```python
from build123d import *

# Parameters (mm, degrees)
SKETCH1_W           = 35
SKETCH1_H           = 10.4
BOSS_EXTRUDE1_DEPTH = 1
BOSS_EXTRUDE3_DEPTH = 3
SKETCH3_W           = 3.5
SKETCH3_H           = 8.5
BOSS_EXTRUDE4_DEPTH = 1.2


with BuildPart() as part:
    # Sketch1 → Boss-Extrude1 (new body)
    with BuildSketch(Plane.XY):
        Rectangle(SKETCH1_W, SKETCH1_H)
    extrude(amount=BOSS_EXTRUDE1_DEPTH)

    # Sketch2 → Boss-Extrude3 (add)
    with BuildSketch(Plane.XY.offset(1)):
        with BuildLine():
            Line((15.253902663, 2.079032558), (10.253902663, 2.079032558))
            ThreePointArc((10.253902663, 2.079032558), (9.003902663, 3.329032558), (10.253902663, 4.579032558))
            Line((10.253902663, 4.579032558), (15.253902663, 4.579032558))
            ThreePointArc((15.253902663, 4.579032558), (16.503902663, 3.329032558), (15.253902663, 2.079032558))
        make_face()
    extrude(amount=BOSS_EXTRUDE3_DEPTH)

    # Sketch3 → Boss-Extrude4 (add)
    with BuildSketch(Plane.XY.offset(1)):
        with Locations((-1.547221583, 0.122630604)):
            Rectangle(SKETCH3_W, SKETCH3_H)
    extrude(amount=BOSS_EXTRUDE4_DEPTH)


solid = part.part
```
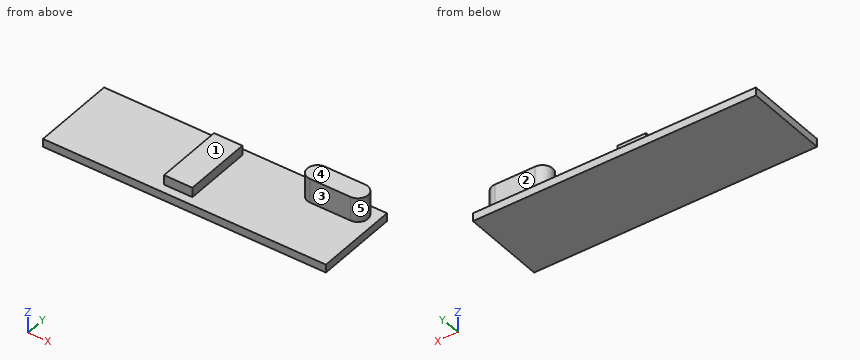
CAD build for the part. Positions are in the model's coordinates, mm. Face numbers are marked on the shaded views. A direction names the side the tool comes from. Round coordinates to 2 decimals unless told otherwise and drop trailing zeros. Write each loop counter-clockwise with the first axis right and the second up, starting at its lowest first coordinate (ties: lowest second). Pieces come first, ordered by that corner, then holes. Notation, with made-up numbers: (60, 38) -> (108, 38) arc R12 ccw to (108, 42) -> close; hole circle Ø7 at (70.5, -13.5). An arc over 180 degrees is marked (long way). Answer in a Markdown table with one row per item. Add a question column.
Item 1: Saw through at C-C, the plane x = 6. Write the cut outline in (y, z), then the cut area to 3 significant figures.
Item 2: Saw through at A-A, the plane z = 1.45. Write the cut outline in (x, y).
Item 3: Saw through at D-D, the plane z = 3.25. Write the cut outline in (x, y), then the cut area to 3 significant figures.
Item 4: Which spindle directions (+Z, -Z, +X, -X, +Y, -Y) get a long thin tool onto all of the face, cutting with end or side? Do the marked faces 1, 2, 3, 4 and 5. Say none if no direction does.
Item 5: Drill centre lines: line 1 (X direction, y = -3.25, z = 1.6); line 2 (Z direction, x = 6, y = 1); line 3 (Y direction, x = 10.5, z = 3.1). Where is each one in solid material? Low to high. Write a range as from..to.
Item 6: Saw through at B-B, the plane y = 0.75. Write the cut outline in (x, z).
Item 7: Drop flat-ended pins along their axis: pin 1 Ø3 at (x, y) = (5.5, 0.5) entering from +Z; pin 2 Ø1 at (x, z) = (-2, 2) entering from -Y; pin 3 Ø0.6 at (y, z) = (2, 1.5) entering from -X. Give the stop position or say it passes through.
Findings below:
| question | item | result |
|---|---|---|
| 1 | outline | (-5.2, 0) -> (5.2, 0) -> (5.2, 1) -> (-5.2, 1) -> close |
| 1 | area | 10.4 mm^2 |
| 2 | outline | (-3.3, -4.13) -> (0.2, -4.13) -> (0.2, 4.37) -> (-3.3, 4.37) -> close; (10.25, 2.08) -> (15.25, 2.08) arc R1.25 ccw to (15.25, 4.58) -> (10.25, 4.58) arc R1.25 ccw to start |
| 3 | outline | (10.25, 2.08) -> (15.25, 2.08) arc R1.25 ccw to (15.25, 4.58) -> (10.25, 4.58) arc R1.25 ccw to start |
| 3 | area | 17.4 mm^2 |
| 4 | face 1 | +Z, -X, +Y, -Y |
| 4 | face 2 | +Z, +X, -X, +Y |
| 4 | face 3 | +Z, +X, -Y |
| 4 | face 4 | +Z, +X, -X, +Y, -Y |
| 4 | face 5 | +Z, +X |
| 5 | line 1 | x = -3.3..0.2 |
| 5 | line 2 | z = 0..1 |
| 5 | line 3 | y = 2.08..4.58 |
| 6 | outline | (-17.5, 0) -> (17.5, 0) -> (17.5, 1) -> (0.2, 1) -> (0.2, 2.2) -> (-3.3, 2.2) -> (-3.3, 1) -> (-17.5, 1) -> close |
| 7 | pin 1 | stops at z = 1 |
| 7 | pin 2 | stops at y = -4.13 |
| 7 | pin 3 | stops at x = -3.3 |
